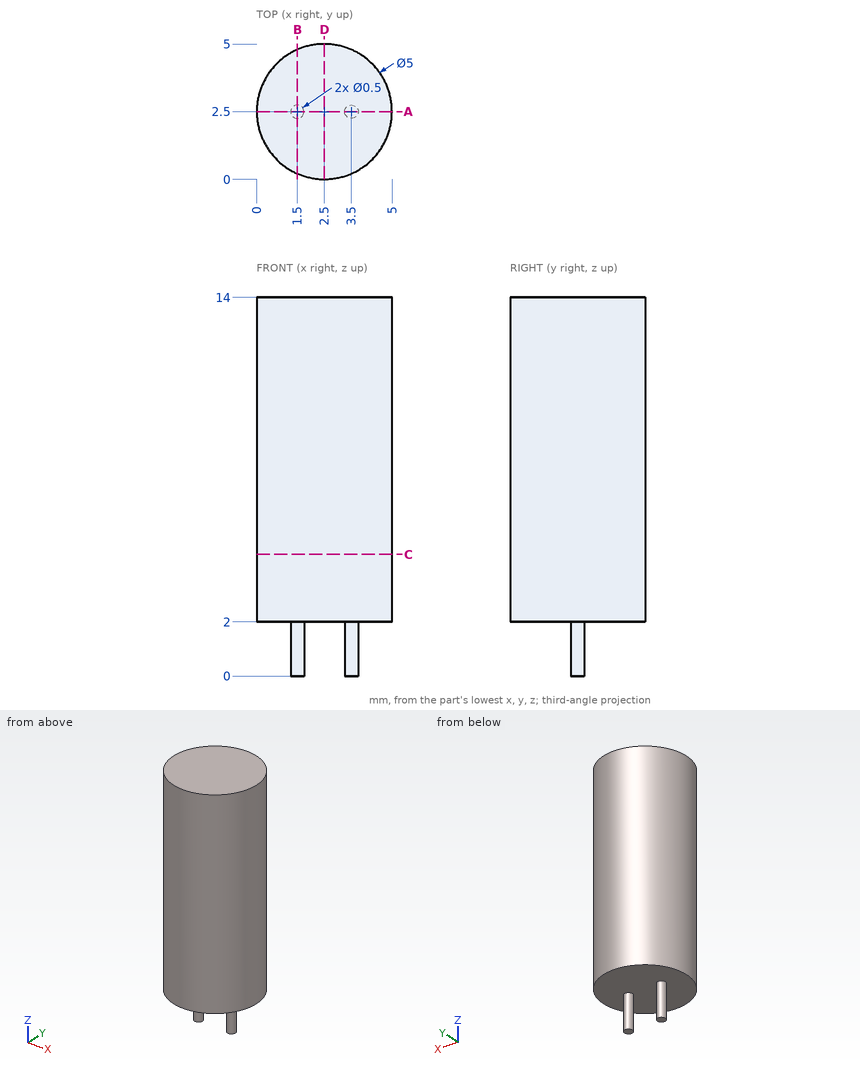
Job drawing, mm, ordinate dimensions from the low corner. One solid piece. Coordinates: 2 decimals unless noted, no trailing zeros. Order: outer loops, then holes, each group sorted by start corner. A loop starts at its lowest first (then second) coordinate and runs counter-clockwise, first axis right, second up. Notation, with made-up numbers: (16.25, 74.25) - (73.25, 74.25) arc R22 cw to (73.25, 110.25) - close; hole circle Ø11 at (67, 85.25). An arc over 180 degrees is marked (long way). Return JSON: item names as keys, results as strings. Group by question number.
1) Flat gauge pins, fed straight in: P1, Ø3, axis at x = 4, z = 2, coming from the +Y side; P2, Ø3, axis at y = 4.5, z = 3.5, coming from the +X side. Where does each tip first touch, or does it go through?
2) Saw through at B-B, the plane x = 1.5. Write the cut outline in (y, z), plus the area to 3 significant figures.
3) Saw through at A-A, the plane y = 2.5. Write the cut outline in (x, z).
4) Saw through at D-D, the plane x = 2.5. Write the cut outline in (y, z).
5) Probe line 1 (Z direction, x = 0.9, y = 1.1); line 2 (Y direction, x = 4.3, z = 13); line 3 (Y direction, x = 4.65, z = 7.75). List the from-to ranges inside material, lowest first. Write a range as from..to.
6) Saw through at C-C, the plane z = 4.5. Write the cut outline in (x, y), plus the area to 3 significant figures.
Values found:
{
 "1": {"P1": "stops at y = 5", "P2": "stops at x = 4.95"},
 "2": {"outline": "(0.21, 2) - (2.25, 2) - (2.25, 0) - (2.75, 0) - (2.75, 2) - (4.79, 2) - (4.79, 14) - (0.21, 14) - close", "area": "56.0 mm²"},
 "3": {"outline": "(0, 2) - (1.25, 2) - (1.25, 0) - (1.75, 0) - (1.75, 2) - (3.25, 2) - (3.25, 0) - (3.75, 0) - (3.75, 2) - (5, 2) - (5, 14) - (0, 14) - close"},
 "4": {"outline": "(0, 2) - (5, 2) - (5, 14) - (0, 14) - close"},
 "5": {"line 1": "z = 2..14", "line 2": "y = 0.77..4.23", "line 3": "y = 1.22..3.78"},
 "6": {"outline": "circle Ø5 at (2.5, 2.5)", "area": "19.6 mm²"}
}
